from build123d import *

# Parameters (mm, degrees)
SKETCH1_W           = 33
SKETCH1_H           = 38
BOSS_EXTRUDE1_DEPTH = 1.6
SKETCH2_R           = 1.65
CUT_EXTRUDE1_DEPTH  = 1.6
SKETCH3_W           = 10
SKETCH3_H           = 7
BOSS_EXTRUDE2_DEPTH = 5.4
SKETCH4_W           = 21.3
SKETCH4_H           = 16
BOSS_EXTRUDE3_DEPTH = 20.5
SKETCH5_W           = 20.5
SKETCH5_H           = 8.3
BOSS_EXTRUDE4_DEPTH = 10


with BuildPart() as part:
    # Sketch1 → Boss-Extrude1 (new body)
    with BuildSketch(Plane(origin=(0, 0, 0), x_dir=(1, 0, 0), z_dir=(0, 1, 0))):
        with Locations((16.5, 19)):
            Rectangle(SKETCH1_W, SKETCH1_H)
    extrude(amount=BOSS_EXTRUDE1_DEPTH)

    # Sketch2 → Cut-Extrude1 (cut)
    with BuildSketch(Plane(origin=(0, 1.6, 0), x_dir=(1, 0, 0), z_dir=(0, 1, 0))):
        with Locations(Location((29.05, 3.95, 0), (0, 0, 270))):
            Circle(SKETCH2_R)
        with Locations(Location((3.95, 3.95, 0), (0, 0, 90))):
            Circle(SKETCH2_R)
        with Locations(Location((29.05, 34.05, 0), (0, 0, 90))):
            Circle(SKETCH2_R)
    extrude(amount=-CUT_EXTRUDE1_DEPTH, mode=Mode.SUBTRACT)

    # Sketch3 → Boss-Extrude2 (add)
    with BuildSketch(Plane(origin=(0, 1.6, 0), x_dir=(1, 0, 0), z_dir=(0, 1, 0))):
        with Locations((16.5, 3.5)):
            Rectangle(SKETCH3_W, SKETCH3_H)
    extrude(amount=BOSS_EXTRUDE2_DEPTH)

    # Sketch4 → Boss-Extrude3 (add)
    with BuildSketch(Plane(origin=(0, 1.6, 0), x_dir=(1, 0, 0), z_dir=(0, 1, 0))):
        with Locations((17.45, 18.6)):
            Rectangle(SKETCH4_W, SKETCH4_H)
    extrude(amount=BOSS_EXTRUDE3_DEPTH)

    # Sketch5 → Boss-Extrude4 (add)
    with BuildSketch(Plane(origin=(0, 1.6, 0), x_dir=(1, 0, 0), z_dir=(0, 1, 0))):
        with Locations((12.85, 33.85)):
            Rectangle(SKETCH5_W, SKETCH5_H)
    extrude(amount=BOSS_EXTRUDE4_DEPTH)


solid = part.part
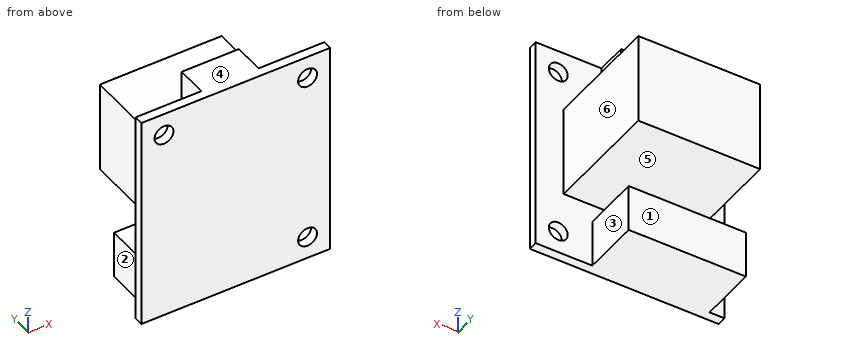
Design review of the part built by this model. Coordinates are the model's own, in mm. Face numbers are marked on the shaded views. A direction names the side the tool comes from. Round coordinates to 2 decimals unless told otherwise and drop trailing zeros. Write each loop counter-clockwise with the first axis right and the second up, starting at its lowest first coordinate (ties: lowest second). Pieces come first, ordered by that corner, then holes.
Item 1: Wall thickness on L1, parallel to Z at x = 12.5, y = 5.25; L2, parallel to X at y = 0.45, z = -3.95; L3, parallel to Y at x = 2, z = -5.5: over which ranges is each line inside the solid? List them lowest first.
Item 2: Consider section A-A on x = 29.05. Give the boundary of the cut face in (y, z).
Item 3: For pin 1 Ø8 at (y, z) = (7.5, -16) entering from -X; pin 2 Ø3 at (y, z) = (10.5, -14) entering from +X; pin 3 Ø2 at (x, z) = (29.05, -3.95) entering from +Y; pin 4 Ø6.5 at (y, z) = (8, -35) entering from -X, all flat-tipped, find the tip position at first contact; note any pin that passes through.
Item 4: Draft analysis for pull direction Z (two halves, no side actions). For the marked faces 4, 5 and 6, state which applies: released by +Z, released by -Z, zero draft, split by the parting line, or undercut.
Item 5: Consider section D-D on x = 3.95. Give the boundary of the cut face in (y, z), and give its area (3 significant figures).
Item 6: Consider section B-B on z = -34.05. Give the boundary of the cut face in (x, y).
Item 7: Consider section C-C on y = 2.5. Give the boundary of the cut face in (x, z), and give its area (3 significant figures).
Item 8: For the marked faces 1, 2 and 3, list the 3-axis set-ups (+Z, -Z, +X, -X, +Y, -Y) from which the entire face can be reached by the end or side of a thin tool; tool diameter is ignored.
Check values:
1. L1: z = -38 to -29.7, -26.6 to -10.6, -7 to 0
1. L2: x = 0 to 2.3, 5.6 to 27.4, 30.7 to 33
1. L3: y = 0 to 1.6
2. outline: (0, -38) - (1.6, -38) - (1.6, -35.7) - (0, -35.7) - close; (0, -32.4) - (1.6, -32.4) - (1.6, -5.6) - (0, -5.6) - close; (0, -2.3) - (1.6, -2.3) - (1.6, 0) - (0, 0) - close
3. pin 1: stops at x = 6.8
3. pin 2: stops at x = 28.1
3. pin 3: passes through
3. pin 4: stops at x = 2.6
4. face 4: released by +Z
4. face 5: undercut
4. face 6: zero draft
5. outline: (0, -38) - (11.6, -38) - (11.6, -29.7) - (1.6, -29.7) - (1.6, -5.6) - (0, -5.6) - close; (0, -2.3) - (1.6, -2.3) - (1.6, 0) - (0, 0) - close
5. area: 139 mm2
6. outline: (0, 0) - (27.4, 0) - (27.4, 1.6) - (23.1, 1.6) - (23.1, 11.6) - (2.6, 11.6) - (2.6, 1.6) - (0, 1.6) - close; (30.7, 0) - (33, 0) - (33, 1.6) - (30.7, 1.6) - close
7. outline: (2.6, -38) - (23.1, -38) - (23.1, -29.7) - (2.6, -29.7) - close; (6.8, -26.6) - (28.1, -26.6) - (28.1, -10.6) - (6.8, -10.6) - close; (11.5, -7) - (21.5, -7) - (21.5, 0) - (11.5, 0) - close
7. area: 581 mm2
8. face 1: -Z, +X, -X, +Y
8. face 2: +Z, -Z, -X, +Y
8. face 3: -Z, +X, +Y
